Check sheet for the drawn part. Datum: minimum x, y, z corner. Units: mm. Give positions to 0.01 mm unless a question says otherwise; leave off trailing zeros. Loops run counter-clockwise (first coordinate to the right, second up) from the corner with the lowest first, then second, coordinate; pieces in that order, holes last.
1. Release check for a two-part mould opening along Y. For the marked faces 1, 2 and 3 record: +Y half, -Y half, draft (parallel to the pull), parting line (faces both ways), or undercut.
2. Cross-section at D-D, the plane z = 25.5. Record the cut outline in (x, y), plus the area to 4 significant figures.
3. Material ranges on L1, parallel to Y at x = 26.95, z = 14; L2, parallel to X at y = 13.75, z = 14.5; L3, parallel to Z at x = 22.25, y = 3, recorded low to high.
4. Cross-section at A-A, the plane y = 14. Record the cut outline in (x, z), plus the area to 3 significant figures.
5. Go/stop test with a flat-tipped pin: pin 1 Ø1.8 at (y, z) = (13.5, 13) entering from +X. Record where the tip stops, or that it passes through.
6. Cross-section at B-B, the plane x = 16.5. Record the cut outline in (y, z).
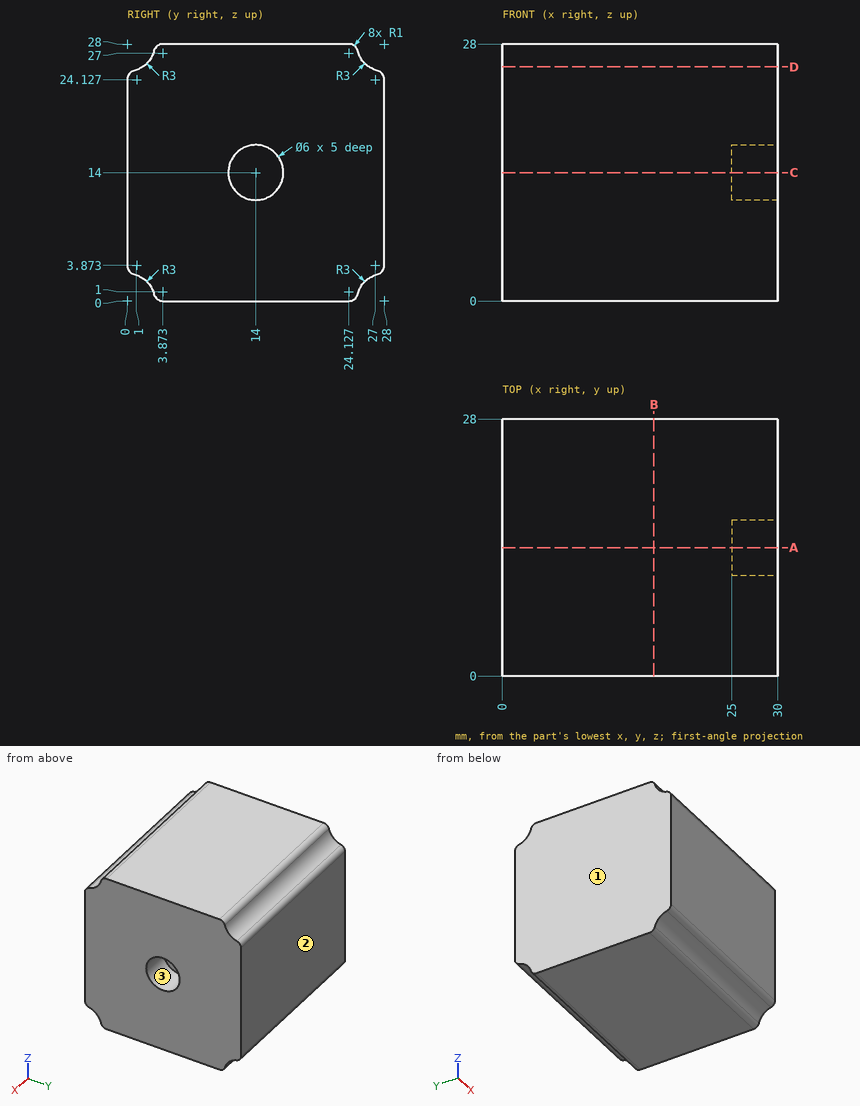
Result:
1. face 1: draft
1. face 2: +Y half
1. face 3: undercut
2. outline: (0, 1.66) - (30, 1.66) - (30, 26.34) - (0, 26.34) - close
2. area: 740.5 mm2
3. L1: y = 0 to 11, 17 to 28
3. L2: x = 0 to 25
3. L3: z = 0.51 to 27.49
4. outline: (0, 0) - (30, 0) - (30, 11) - (25, 11) - (25, 17) - (30, 17) - (30, 28) - (0, 28) - close
4. area: 810 mm2
5. pin 1: stops at x = 25
6. outline: (0, 3.87) arc R1 ccw to (0.75, 2.9) arc R3 cw to (2.9, 0.75) arc R1 ccw to (3.87, 0) - (24.13, 0) arc R1 ccw to (25.1, 0.75) arc R3 cw to (27.25, 2.9) arc R1 ccw to (28, 3.87) - (28, 24.13) arc R1 ccw to (27.25, 25.1) arc R3 cw to (25.1, 27.25) arc R1 ccw to (24.13, 28) - (3.87, 28) arc R1 ccw to (2.9, 27.25) arc R3 cw to (0.75, 25.1) arc R1 ccw to (0, 24.13) - close
